Model file for the job. Use its own axes, mm. Face numbers are marked on the shaded views. A direction names the side the tool comes from. Coordinates: 2 decimals unless noted, no trailing zeros. Write each loop counter-clockwise with the first axis right and the second up, starting at its lowest first coordinate (ties: lowest second). Pieces come first, ordered by that corner, then holes. Notation, with made-up numbers: M 26,72.5 L 77,72.5 A9 ccw 77,77.5 Z; hole C 64,-6 d6. An arc over 180 degrees is marked long. Put each result on its own line as item: value. Start each with the question number.
Q1. Cut at D-D (x = 3.5). Write the cut outline in (y, z), then the cut area to 3 significant figures.
Q2. Drop flat-ended pins along their axis: pin 1 (3 mm diameter, centred on x = 4.5, z = -8, fed in from -Y); pin 2 (2 mm diameter, centred on x = 1, y = 4.5, fed in from -Z); pin 3 (1.8 mm diameter, centred on x = -3.05, z = -9, fed in from -Y); pin 4 (1.8 mm diameter, centred on x = -3.5, y = 4, fed in from -Z). Give the stop position or say it passes through.
Q3. Cut at A-A (y = 6.75). Write the cut outline in (x, z) (3 decimals), then the cut area to 3 significant figures.
Q4. Cut at C-C (z = 9). Write the cut outline in (x, y), then the cut area to 3 significant figures.
Q5. Cut at B-B (x = -3.05). Write the cut outline in (y, z), then the cut area to 3 significant figures.
Q6. Drill centre lines: line 1 along X through (y, z) = (0.5, 9); line 2 along Z through (x, y) = (-2, 4); line 3 along Z through (x, y) = (-1.25, 5.75). Where is each one in solid material? Low to high.
Q7. Pull direction X, two halves, no side cores. Call the marked faces 4, 5 and 6: pulls with the +X half, pulls with the -X half, needs draft (parallel to the pull), parting line crosses it, or undercut.
Q8. Which spindle directions (+Z, -Z, +X, -X, +Y, -Y) get a long thin tool onto all of the face, cutting with end or side? Do the marked faces 1, 2 and 3. Say none if no direction does.
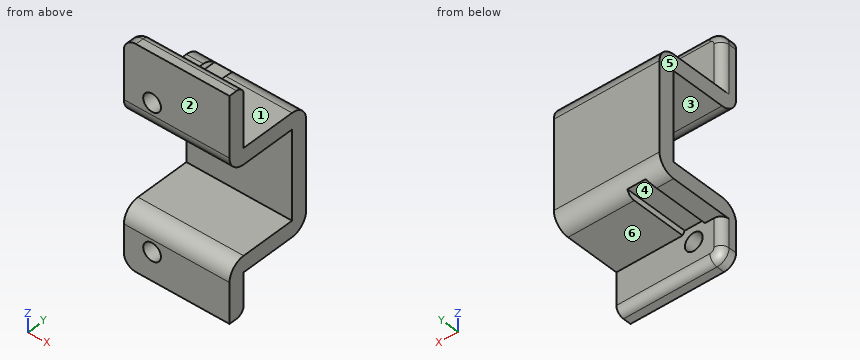
```python
from build123d import *

# Parameters (mm, degrees)
BOSS_EXTRUDE1_DEPTH = 6.55
CUT_EXTRUDE1_REACH  = 20.607
SKETCH2_R           = 1.1
CUT_EXTRUDE2_REACH  = 20.607
FILLET1_R           = 2
FILLET3_R           = 1.5
FILLET4_R           = 1


with BuildPart() as part:
    # Sketch1 → Boss-Extrude1 (new, symmetric)
    with BuildSketch(Plane(origin=(0, 0, 0), x_dir=(0, 0, -1), z_dir=(1, 0, 0))):
        Polygon((-5.5, 8.85), (5.5, 8.85), (5.5, 0), (12.5, 0), (12.5, 2), (7.5, 2), (7.5, 10.85), (-7.5, 10.85), (-7.5, 2), (-15, 2), (-15, 0), (-5.5, 0), align=None)
    extrude(amount=BOSS_EXTRUDE1_DEPTH, both=True)

    # Sketch2 → Cut-Extrude1 (cut, up to next)
    with BuildSketch(Plane(origin=(0, 2, 0), x_dir=(1, 0, 0), z_dir=(0, 1, 0)), mode=Mode.PRIVATE) as cut_extrude1_sk1:
        with Locations(Location((-3.05, -9, 0), (0, 0, 270))):
            Circle(SKETCH2_R)
    cut_extrude1_tool1 = extrude(cut_extrude1_sk1.sketch, amount=-CUT_EXTRUDE1_REACH, mode=Mode.PRIVATE) & part.part
    cut_extrude1 = cut_extrude1_tool1.solids().sort_by_distance((-3.05, 2, 9))[0]
    add(cut_extrude1, mode=Mode.SUBTRACT)

    # Sketch3 → Cut-Extrude2 (cut, up to next)
    with BuildSketch(Plane(origin=(0, 2, 0), x_dir=(1, 0, 0), z_dir=(0, 1, 0)), mode=Mode.PRIVATE) as cut_extrude2_sk1:
        Polygon((-5.3, -9), (-4.175, -10.948557159), (-1.925, -10.948557159), (-0.8, -9), (-1.925, -7.051442841), (-4.175, -7.051442841), align=None)
    cut_extrude2_tool1 = extrude(cut_extrude2_sk1.sketch, amount=CUT_EXTRUDE2_REACH, mode=Mode.PRIVATE) & part.part
    cut_extrude2 = cut_extrude2_tool1.solids().sort_by_distance((-3.05, 2, 9))[0]
    add(cut_extrude2, mode=Mode.SUBTRACT)

    # Mirror1: Cut-Extrude1, Cut-Extrude2 across plane
    add(cut_extrude1.mirror(Plane.XY), mode=Mode.SUBTRACT)
    add(cut_extrude2.mirror(Plane.XY), mode=Mode.SUBTRACT)

    # Fillet1
    # the kernel refuses this fillet: 2 mm, written as the material it takes off along each edge
    with BuildSketch(Plane(origin=(-11.55, 0, -5.5), x_dir=(0, 1, 0), z_dir=(1, 0, 0)), Plane(origin=(11.55, 0, 5.5), x_dir=(0, 1, 0), z_dir=(-1, 0, 0))) as fillet1_piece_1:
        with BuildLine():
            CenterArc((FILLET1_R, -FILLET1_R), FILLET1_R, 90, 90)
            Line((0, -FILLET1_R), (0, 0))
            Line((0, 0), (FILLET1_R, 0))
        make_face()
    extrude(amount=23.1, mode=Mode.SUBTRACT)
    with BuildSketch(Plane(origin=(-6.666025404, 10.85, 7.5), x_dir=(0, 0, -1), z_dir=(1, 0, 0))) as fillet1_piece_2:
        with BuildLine():
            CenterArc((FILLET1_R, -FILLET1_R), FILLET1_R, 90, 90)
            Line((0, -FILLET1_R), (0, 0))
            Line((0, 0), (FILLET1_R, 0))
        make_face()
    extrude(amount=18.216025404, mode=Mode.SUBTRACT)
    with BuildSketch(Plane(origin=(-6.666025404, 10.85, -7.5), x_dir=(0, 0, 1), z_dir=(1, 0, 0))) as fillet1_piece_3:
        with BuildLine():
            CenterArc((FILLET1_R, FILLET1_R), FILLET1_R, 180, 90)
            Line((0, FILLET1_R), (0, 0))
            Line((0, 0), (FILLET1_R, 0))
        make_face()
    extrude(amount=18.216025404, mode=Mode.SUBTRACT)

    # Fillet3
    fillet3_edges = [part.edges().sort_by_distance(p)[0] for p in [
        (-6.55, 1, -12.5),
        (-6.55, 1, 15),
    ]]
    fillet(fillet3_edges, radius=FILLET3_R)

    # Fillet4
    fillet4_edges = [part.edges().sort_by_distance(p)[0] for p in [
        (-6.110660172, 2, 14.560660172),
        (-6.110660172, 2, -12.060660172),
        (-6.55, 2, 10.5),
        (-6.55, 2, -9.25),
        (0.75, 2, -12.5),
        (0.75, 2, 15),
    ]]
    fillet(fillet4_edges, radius=FILLET4_R)


solid = part.part
```
Computed values:
1. outline: M 0,-12.5 L 1,-12.5 A1 ccw 2,-11.5 L 2,-7.5 L 8.85,-7.5 A2 ccw 10.85,-5.5 L 10.85,5.5 A2 ccw 8.85,7.5 L 2,7.5 L 2,14 A1 ccw 1,15 L 0,15 L 0,7.5 A2 ccw 2,5.5 L 8.85,5.5 L 8.85,-5.5 L 2,-5.5 A2 ccw 0,-7.5 Z
1. area: 86.5 mm2
2. pin 1: y = 0
2. pin 2: z = -7.5
2. pin 3: through
2. pin 4: z = -7.44
3. outline: M -6.55,-7.5 L -4.434,-7.5 L -4.175,-7.051 L -1.925,-7.051 L -1.666,-7.5 L 6.55,-7.5 L 6.55,-5.5 L -6.55,-5.5 Z; M -6.55,5.5 L 6.55,5.5 L 6.55,7.5 L -1.666,7.5 L -1.925,7.051 L -4.175,7.051 L -4.434,7.5 L -6.55,7.5 Z
3. area: 50.1 mm2
4. outline: M -6.55,0 L -4.15,0 L -4.15,2 L -5.55,2 A1 ccw -6.55,1 Z; M -1.95,0 L 6.55,0 L 6.55,2 L -1.95,2 Z
4. area: 21.6 mm2
5. outline: M 0,-12.5 L 1,-12.5 A1 ccw 2,-11.5 L 2,-10.1 L 0,-10.1 Z; M 0,-7.9 L 2,-7.9 L 2,-7.05 L 10.11,-7.05 A2 ccw 10.85,-5.5 L 10.85,5.5 A2 ccw 10.11,7.05 L 2,7.05 L 2,7.9 L 0,7.9 L 0,7.5 A2 ccw 2,5.5 L 8.85,5.5 L 8.85,-5.5 L 2,-5.5 A2 ccw 0,-7.5 Z; M 0,10.1 L 2,10.1 L 2,14 A1 ccw 1,15 L 0,15 Z
5. area: 70.8 mm2
6. line 1: -6.55 to -4.15, -1.95 to 6.55
6. line 2: -7.05 to -5.5, 5.5 to 7.05
6. line 3: -7.5 to -5.5, 5.5 to 7.5
7. face 4: undercut
7. face 5: pulls with the -X half
7. face 6: needs draft
8. face 1: +Z, +X, -X, +Y
8. face 2: +Z, -Z, +X, -X, -Y
8. face 3: +X, -X, -Y
